from build123d import *

# Parameters (mm, degrees)
BOSS_EXTRUDE1_DEPTH = 30


with BuildPart() as part:
    # Sketch3 → Boss-Extrude1 (new body)
    with BuildSketch(Plane(origin=(0, 0, 0), x_dir=(0, 0, -1), z_dir=(1, 0, 0))):
        with BuildLine():
            Line((-2, 22.226110771), (-2, 12.821942467))
            Line((-2, 12.821942467), (-4.678920426, 12.104127903))
            Line((-4.678920426, 12.104127903), (-9.381004578, 20.248376555))
            ThreePointArc((-9.381004578, 20.248376555), (-9.496151336, 21.498457721), (-8.620764237, 22.398268325))
            ThreePointArc((-8.620764237, 22.398268325), (-6.211657082, 23.182219831), (-3.733333333, 23.707851489))
            ThreePointArc((-3.733333333, 23.707851489), (-2.525320566, 23.366286196), (-2, 22.226110771))
        make_face()
    extrude(amount=BOSS_EXTRUDE1_DEPTH)


solid = part.part
Build history of the part. All positions in model axes, mm. Round coordinates to 2 decimals unless told otherwise and drop trailing zeros. Write each loop counter-clockwise with the first axis right and the second up, starting at its lowest first coordinate (ties: lowest second). Pieces come first, ordered by that corner, then holes. Notation, with made-up numbers: M 84.5,10.25 L 108.5,10.25 A15 cw 108.5,17.25 Z; hole C 62.25,34 d4. An arc over 180 degrees is marked long. Answer in a Markdown table with one row per item.
1. Flat gauge pins, fed straight in: P1, Ø2, axis at x = 22.5, y = 15, coming from the +Z side; P2, Ø1, axis at x = 10, y = 13.5, coming from the +Z side; P3, Ø1.5, axis at x = 10, y = 13.5, coming from the +Z side. Where does each tip first touch, or does it go through?
Geometry check:
| item | result |
|---|---|
| P1 | z = 6.93 |
| P2 | z = 5.77 |
| P3 | z = 5.92 |
2. Saw through at A-A (x = 10.5). List the corners of the cut face in (y, z).
Geometry check:
| item | result |
|---|---|
| outline | M 12.1,4.68 L 12.82,2 L 22.23,2 A1.5 ccw 23.71,3.73 A24 ccw 22.4,8.62 A1.5 ccw 20.25,9.38 Z |
3. Probe L1, parallel to Y at x = 4.5, z = 6; L2, parallel to Z at x = 24.25, y = 19; L3, parallel to Y at x = 19.5, z = 6.75. List the from-to ranges inside material, lowest first. Write a range as [from, to].
Geometry check:
| item | result |
|---|---|
| L1 | [14.39, 23.24] |
| L2 | [2, 8.66] |
| L3 | [15.69, 23.03] |
4. Saw through at B-B (z = 9). List the corners of the cut face in (x, y), and give its area (3 significant figures).
Geometry check:
| item | result |
|---|---|
| outline | M 0,19.59 L 30,19.59 L 30,22.18 L 0,22.18 Z |
| area | 77.9 mm2 |
5. Saw through at C-C (y = 15). List the corners of the cut face in (x, z), and give its area (3 significant figures).
Geometry check:
| item | result |
|---|---|
| outline | M 0,2 L 30,2 L 30,6.35 L 0,6.35 Z |
| area | 131 mm2 |
